Read the model definition and answer for the solid it produces. Units are mm, in the model's axes. A direction names the side the tool comes from. Give positions to 0.01 mm unless a question says otherwise; leave off trailing zeros. Loops run counter-clockwise (first coordinate to the right, second up) from the corner with the lowest first, then second, coordinate; pieces in that order, holes last. Notation, with made-up numbers: (69, -36.75) - (128, -36.75) arc R20 ccw to (128, -31.75) - close; hole circle Ø8 at (-20.5, -11.75). An arc over 180 degrees is marked (long way). Write item = value, one per line.
Autodesk Inventor part; units mm, degrees
ref_plane "Work Plane1" through (-11.2547, -6.35, -50.8) normal (-1, 0, 0) x (0, 0, 1)
ref_plane "YZ Plane" through (0, 0, 0) normal (1, 0, 0) x (0, 1, 0)
ref_plane "XZ Plane" through (0, 0, 0) normal (0, 1, 0) x (-1, 0, 0)
sketch "Sketch1" plane through (0, 0, 0) normal (0, 1, 0) x (-1, 0, 0)
  line L0 (11.2547, 50.8) -> (-11.2547, 50.8)
  line L1 (-11.2547, 50.8) -> (-11.2547, -50.8)
  line L2 (-11.2547, -50.8) -> (11.2547, -50.8)
  line L3 (11.2547, -50.8) -> (11.2547, 50.8)
  line L4 (11.2547, 50.8) -> (-11.2547, -50.8) construction
  line L5 (-11.2547, 50.8) -> (11.2547, -50.8) construction
  point P0 (0, 0)
  dimension "d0" = 101.6
  dimension "d1" = 22.5095
extrude "Extrusion1" add sketch "Sketch1" against normal blind 6.35
sketch "Sketch2" plane through (0, 0, 0) normal (0, 1, 0) x (1, 0, 0)
  line L0 (11.2547, -50.8) -> (-11.2547, -50.8)
  line L1 (-11.2547, 50.8) -> (11.2547, 50.8)
  line L2 (-11.2547, -50.8) -> (-4.9047, -50.8)
  line L3 (-4.9047, -50.8) -> (-4.9047, 50.8)
  line L4 (-4.9047, 50.8) -> (-11.2547, 50.8)
  line L5 (-11.2547, 50.8) -> (-11.2547, -50.8)
  point P0 (0, 0)
  dimension "d4" = 6.35
extrude "Extrusion2" add sketch "Sketch2" along normal blind 76.2
sketch "Sketch4" plane through (0, 0, 0) normal (0, 1, 0) x (1, 0, 0)
  line L0 (-4.9047, -50.8) -> (11.2547, -50.8) construction
  line L1 (3.175, -50.8) -> (3.175, 50.8) construction
  line L2 (-11.2547, 50.8) -> (11.2547, 50.8) construction
  point P0 (0, 0)
  point P1 (3.175, -38.1)
  point P2 (3.175, -12.7)
  point P3 (3.175, 12.7)
  point P4 (3.175, 38.1)
  dimension "d11" = 12.7
  dimension "d14" = 25.4
hole "Hole1" at (3.175, 0, 38.1) at (3.175, 0, 12.7) at (3.175, 0, -12.7) at (3.175, 0, -38.1) direction (0, -1, 0) diameter 5.1054 end through all
ref_plane "Work Plane1" through (-11.2547, -6.35, -50.8) normal (-1, 0, 0) x (0, 0, 1)
sketch "Sketch7" plane through (-11.2547, -6.35, -50.8) normal (-1, 0, 0) x (0, 0, 1)
  line L0 (0, 6.35) -> (101.6, 6.35)
  line L1 (0, 82.55) -> (101.6, 82.55)
  line L2 (101.6, 0) -> (101.6, 82.55)
  line L3 (0, 0) -> (0, 82.55)
  line L4 (101.6, 6.35) -> (101.6, 82.55)
  line L5 (0, 6.35) -> (101.6, 6.35)
  line L6 (101.6, 6.35) -> (101.6, 82.55)
  line L7 (101.6, 82.55) -> (0, 82.55)
  line L8 (0, 82.55) -> (0, 6.35)
  point P0 (50.8, 6.35)
extrude "Extrusion5" cut sketch "Sketch7" against normal through all
sketch "Sketch8" plane through (-11.2547, -6.35, -50.8) normal (-1, 0, 0) x (0, 0, 1)
  line L0 (0, 0) -> (0, 6.35)
  line L1 (101.6, 0) -> (101.6, 6.35)
  line L2 (101.6, 0) -> (0, 0)
  line L3 (0, 0) -> (101.6, 0)
  line L4 (101.6, 0) -> (101.6, 76.2)
  line L5 (101.6, 76.2) -> (0, 76.2)
  line L6 (0, 76.2) -> (0, 0)
  point P0 (50.8, 6.35)
  dimension "d51" = 76.2
extrude "Extrusion6" add sketch "Sketch8" along normal blind 6.35
sketch "Sketch9" plane through (-11.2547, -6.35, -50.8) normal (1, 0, 0) x (0, 0, -1)
  line L0 (-101.6, 76.2) -> (0, 76.2)
  line L1 (0, 76.2) -> (0, 0)
  line L2 (-101.6, 0) -> (-101.6, 76.2)
  line L3 (0, 0) -> (-101.6, 0)
  line L4 (-76.2, 63.5) -> (-76.2, 19.05) construction
  line L5 (-79.5782, 63.5) -> (-79.5782, 19.05)
  line L6 (-72.8218, 19.05) -> (-72.8218, 63.5)
  arc A0 (-72.8218, 63.5) -> (-79.5782, 63.5) centre (-76.2, 63.5) ccw
  arc A1 (-79.5782, 19.05) -> (-72.8218, 19.05) centre (-76.2, 19.05) ccw
  line L7 (-101.6, 63.5) -> (0, 63.5) construction
  line L8 (-101.6, 19.05) -> (0, 19.05) construction
  line L9 (-50.8, 63.5) -> (-50.8, 19.05) construction
  line L10 (-54.1782, 63.5) -> (-54.1782, 19.05)
  line L11 (-47.4218, 19.05) -> (-47.4218, 63.5)
  arc A2 (-47.4218, 63.5) -> (-54.1782, 63.5) centre (-50.8, 63.5) ccw
  arc A3 (-54.1782, 19.05) -> (-47.4218, 19.05) centre (-50.8, 19.05) ccw
  line L12 (-25.4, 63.5) -> (-25.4, 19.05) construction
  line L13 (-28.7782, 63.5) -> (-28.7782, 19.05)
  line L14 (-22.0218, 19.05) -> (-22.0218, 63.5)
  arc A4 (-22.0218, 63.5) -> (-28.7782, 63.5) centre (-25.4, 63.5) ccw
  arc A5 (-28.7782, 19.05) -> (-22.0218, 19.05) centre (-25.4, 19.05) ccw
  point P0 (-50.8, 6.35)
  point P1 (-76.2, 41.275)
  point P2 (-50.8, 41.275)
  point P3 (-25.4, 41.275)
  dimension "d54" = 25.4
  dimension "d55" = 12.7
  dimension "d56" = 19.05
  dimension "d58" = 6.7564
  dimension "d59" = 25.4
extrude "Extrusion7" cut sketch "Sketch9" against normal through all contours A0 L6 A1 L5 | A2 L11 A3 L10 | A4 L14 A5 L13
equation "\"d0\" = BaseLength"
equation "\"d1\" = BaseWidth"
equation "\"d2\" = BaseThickness"
equation "\"d4\" = BackWidth"
equation "\"d5\" = BackHeight"
equation "\"d54\" = deltaForSlots"
equation "\"BaseWidth\" = 22.50948"
equation "\"BaseLength\" = 101.6"
equation "\"BaseThickness\" = 6.35"
equation "\"BackWidth\" = 6.35"
equation "\"BackHeight\" = 76.2"
equation "\"TopBackExtension\" = 50.8"
equation "\"TopFrontExtension\" = 50.8"
equation "\"TopThickness\" = 6.35"
equation "\"offsetForFirstHole\" = 12.7"
equation "\"holeSpacingForMotorBracket\" = 76.2"
equation "\"offsetForBracketHoleFromEdge\" = 6.35"
equation "\"holeSpacingForVariationInMotorBracketHoles\" = 19.05"
equation "\"deltaForSlots\" = 0.25 * BaseLength"
properties part number "pullyBracketLowerPortion" material "PC/ABS Plastic"
1) Find the intervals of material crossed by probe 1 along Z at (x, y) = (-15.5, 56); probe 2 along X at (y, z) = (-1, 38); probe 3 along Z at (x, y) = (1, -0.5), in increasing order.
Output:
probe_1 = -50.8 to -28.78, -22.02 to -3.38, 3.38 to 22.02, 28.78 to 50.8
probe_2 = -17.6 to 0.62, 5.73 to 11.25
probe_3 = -50.8 to -39.44, -36.76 to -14.04, -11.36 to 11.36, 14.04 to 36.76, 39.44 to 50.8
2) Each of these flat-tipped pins is pushed along its axis until it touches: P1, Ø1.5, axis at x = 0, z = 10, coming from the +Y side; P2, Ø8, axis at x = 3.175, z = -38.1, coming from the -Y side; P3, Ø4, axis at x = 3.175, z = 38.1, coming from the +Y side; P4, Ø12, axis at y = 18, z = -9, coming from the +X side. Where does it stop, or does it pass through?
Output:
P1 = 0
P2 = -6.35
P3 = through
P4 = -11.25
3) A cutting plane is placed at C-C on z = 44. Determine the outline of the cut face in (x, y), then the cut area to 3 significant figures.
Output:
outline = (-17.6, -6.35) - (11.25, -6.35) - (11.25, 0) - (-11.25, 0) - (-11.25, 69.85) - (-17.6, 69.85) - close
area = 627 mm²
4) A cutting plane is placed at D-D on z = 12.7. Determine the outline of the cut face in (x, y).
Output:
outline = (-17.6, -6.35) - (0.62, -6.35) - (0.62, 0) - (-11.25, 0) - (-11.25, 69.85) - (-17.6, 69.85) - close; (5.73, -6.35) - (11.25, -6.35) - (11.25, 0) - (5.73, 0) - close
5) A cutting plane is placed at B-B on y = 30.5. Determine the outline of the cut face in (x, z), then the cut area to 3 significant figures.
Output:
outline = (-17.6, -50.8) - (-11.25, -50.8) - (-11.25, -28.78) - (-17.6, -28.78) - close; (-17.6, -22.02) - (-11.25, -22.02) - (-11.25, -3.38) - (-17.6, -3.38) - close; (-17.6, 3.38) - (-11.25, 3.38) - (-11.25, 22.02) - (-17.6, 22.02) - close; (-17.6, 28.78) - (-11.25, 28.78) - (-11.25, 50.8) - (-17.6, 50.8) - close
area = 516 mm²
6) A tool of negligible diameter and unlimited length cuts with its end or side. For faces 4 (the face through (-14, 35, 28.778)), 5 (the face through (4.15, -3.22, 15.06)), 6 (the face through (0, 0, -1)), from which of +Z, -Z, +X, -X, +Y, -Y can it reach the whole face along a straight path? Write none if from no direction.
Output:
face_4 = +X, -X
face_5 = +Y, -Y
face_6 = +Z, -Z, +X, +Y
7) A cutting plane is placed at A-A on z = 0. Determine the outline of the cut face in (x, y), then the cut area to 3 significant figures.
Output:
outline = (-17.6, -6.35) - (11.25, -6.35) - (11.25, 0) - (-11.25, 0) - (-11.25, 9.32) - (-17.6, 9.32) - close; (-17.6, 60.53) - (-11.25, 60.53) - (-11.25, 69.85) - (-17.6, 69.85) - close
area = 302 mm²
8) The mould has two halves that part along Z. Classify faces 1 (the face through (-17.605, 32, 11)), 2 (the face through (-12, 23, -50.8)), 3 (the face through (2.408, -3.219, 40.535)): pulls with the +Z half, pulls with the -Z half, needs draft (parallel to the pull), parting line crosses it, or undercut.
Output:
face_1 = needs draft
face_2 = pulls with the -Z half
face_3 = undercut
